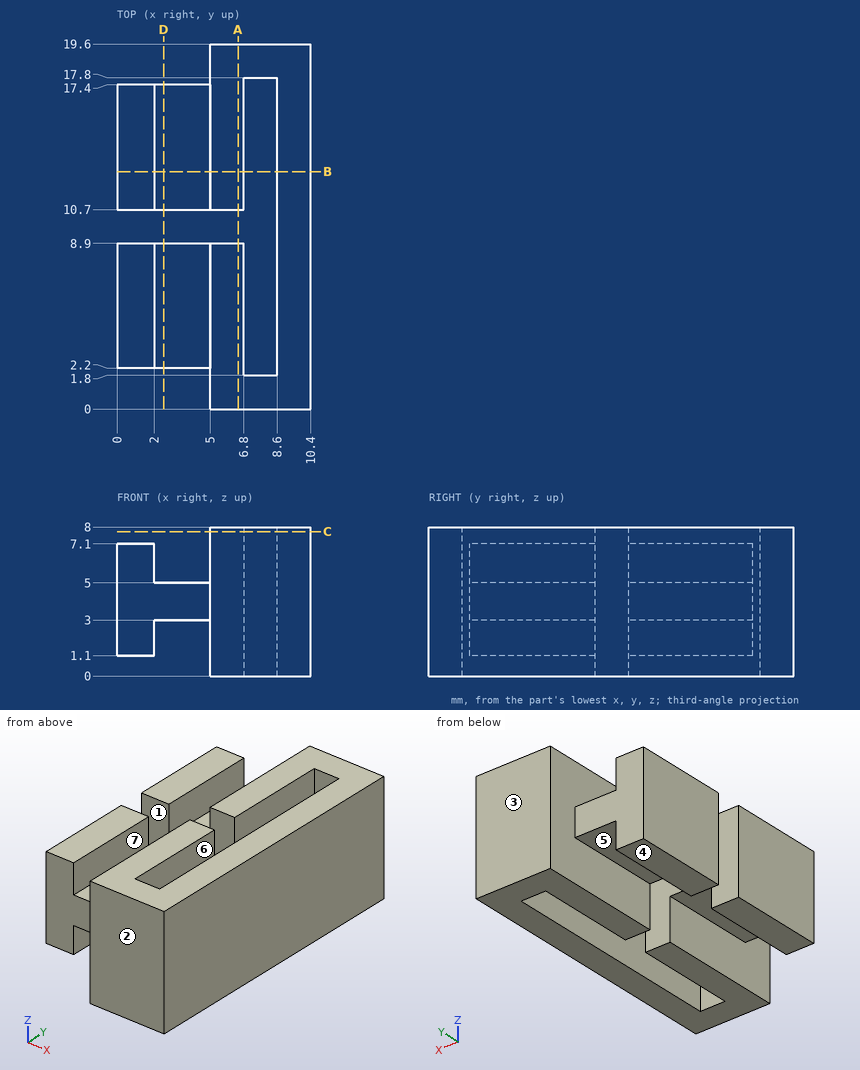
Answer from the drawing. Dimensions are ordinates in mm from the lowest x, y and z of the part. A direction names the side the tool comes from. Give positions to 0.01 mm unless a question says otherwise; leave off trailing zeros. Order: outer loops, then holes, each group sorted by start corner. A loop starts at its lowest first (then second) coordinate and runs counter-clockwise, first axis right, second up. Notation, with made-up numbers: (67, 73.25) - (82, 73.25) arc R5 ccw to (82, 81.25) - close; hole circle Ø6 at (-30, 25.25). An arc over 180 degrees is marked (long way). One line per item, written item: value. Start each with the question number.
1. Each of these flat-tipped pins is pushed along its axis until it touches: pin 1 Ø1.5 at (x, z) = (1.5, 3.5) entering from -Y; pin 2 Ø1.5 at (x, y) = (3, 12) entering from +Z; pin 3 Ø0.9 at (x, y) = (4, 4) entering from -Z. Where does it stop, or does it pass through?
2. For a pull along Y with two mould halves and no side action, classify the marked faces 1, 2, 3 and 4 as released by +Y, released by -Y, zero draft, split by the parting line, or undercut.
3. Which of the six approach directions +Z, -Z, +X, -X, +Y, -Y give full straight-line access (tool end or side, diameter ignored) to the marked faces 5, 6 and 7?
4. Section C-C, the plane z = 7.75 is taken. Write down the section's boundary in (x, y), then the cut area to 3 significant figures.
5. Section D-D, the plane x = 2.5 is taken. Write down the section's boundary in (y, z), then the cut area to 3 significant figures.
6. Section A-A, the plane x = 6.5 is taken. Write down the section's boundary in (y, z), then the cut area to 3 significant figures.
7. Section B-B, the plane y = 12.75 is taken. Write down the section's boundary in (x, z), then the cut area to 3 significant figures.
8. Consider line 1 (X direction, y = 3.75, z = 1.25); line 2 (X direction, y = 2.25, z = 3.25); line 3 (Y direction, x = 3.75, z = 4). Determine where each line is inside the solid, lowest interval first.
Filled sheet:
1. pin 1: y = 2.2
1. pin 2: z = 5
1. pin 3: z = 3
2. face 1: undercut
2. face 2: released by -Y
2. face 3: released by +Y
2. face 4: zero draft
3. face 5: -Z, +Y, -Y
3. face 6: +Z, -Z
3. face 7: +Z, +Y, -Y
4. outline: (5, 0) - (10.4, 0) - (10.4, 19.6) - (5, 19.6) - (5, 10.7) - (6.8, 10.7) - (6.8, 17.8) - (8.6, 17.8) - (8.6, 1.8) - (6.8, 1.8) - (6.8, 8.9) - (5, 8.9) - close
4. area: 73.8 mm²
5. outline: (2.2, 3) - (8.9, 3) - (8.9, 5) - (2.2, 5) - close; (10.7, 3) - (17.4, 3) - (17.4, 5) - (10.7, 5) - close
5. area: 26.8 mm²
6. outline: (0, 0) - (8.9, 0) - (8.9, 8) - (0, 8) - close; (10.7, 0) - (19.6, 0) - (19.6, 8) - (10.7, 8) - close
6. area: 142 mm²
7. outline: (0, 1.1) - (2, 1.1) - (2, 3) - (5, 3) - (5, 0) - (6.8, 0) - (6.8, 8) - (5, 8) - (5, 5) - (2, 5) - (2, 7.1) - (0, 7.1) - close; (8.6, 0) - (10.4, 0) - (10.4, 8) - (8.6, 8) - close
7. area: 46.8 mm²
8. line 1: 0 to 2, 5 to 6.8, 8.6 to 10.4
8. line 2: 0 to 6.8, 8.6 to 10.4
8. line 3: 2.2 to 8.9, 10.7 to 17.4
